from build123d import *

# Parameters (mm, degrees)
SKETCH_1_R          = 23
SKETCH_1_R_2        = 20
EXTRUDE_1_DEPTH     = 51.2
SKETCH_2_R          = 50
SKETCH_2_R_2        = 23
EXTRUDE_2_DEPTH     = 36
EXTRUDE_3_DEPTH     = 15
SKETCH_4_R          = 8
CUT_EXTRUDE_1_DEPTH = 15
SKETCH_5_W          = 2
SKETCH_5_H          = 10
SKETCH_6_R          = 30
CUT_EXTRUDE_2_DEPTH = 2


with BuildPart() as part:
    # Sketch 1 → Extrude 1 (new body)
    with BuildSketch(Plane.XY):
        Circle(SKETCH_1_R)
        Circle(SKETCH_1_R_2, mode=Mode.SUBTRACT)
    extrude(amount=EXTRUDE_1_DEPTH)

    # Sketch 2 → Extrude 2 (add)
    with BuildSketch(Plane.XY):
        Circle(SKETCH_2_R)
        Circle(SKETCH_2_R_2, mode=Mode.SUBTRACT)
    extrude(amount=EXTRUDE_2_DEPTH)

    # Sketch 3 → Extrude 3 (add)
    with BuildSketch(Plane.XY):
        with BuildLine():
            Line((-43.886196735, -23.958333333), (-13.604720988, -79.427083333))
            ThreePointArc((-13.604720988, -79.427083333), (0, -87.5), (13.604720988, -79.427083333))
            Line((13.604720988, -79.427083333), (43.886196735, -23.958333333))
            ThreePointArc((43.886196735, -23.958333333), (0, -50), (-43.886196735, -23.958333333))
        make_face()
        with BuildLine():
            Line((-13.604720988, 79.427083333), (-43.886196735, 23.958333333))
            ThreePointArc((-43.886196735, 23.958333333), (0, 50), (43.886196735, 23.958333333))
            Line((43.886196735, 23.958333333), (13.604720988, 79.427083333))
            ThreePointArc((13.604720988, 79.427083333), (0, 87.5), (-13.604720988, 79.427083333))
        make_face()
    extrude(amount=EXTRUDE_3_DEPTH)

    # Sketch 4 → Cut-Extrude 1 (cut)
    with BuildSketch(Plane.XY):
        with Locations((0, 72)):
            Circle(SKETCH_4_R)
        with Locations((0, -72)):
            Circle(SKETCH_4_R)
    extrude(amount=CUT_EXTRUDE_1_DEPTH, mode=Mode.SUBTRACT)

    # Sketch 5 → Revolve 1 (revolve)
    with BuildSketch(Plane(origin=(0, 0, 0), x_dir=(0, 0, 1), z_dir=(-0.7071067811865488, 0.7071067811865462, 0)), mode=Mode.PRIVATE) as revolve_1_sk:
        with Locations((19, 52)):
            Rectangle(SKETCH_5_W, SKETCH_5_H)
    revolve(revolve_1_sk.sketch.rotate(Axis((-701.140256875, -701.140256875, 18), (0.7071067811865462, 0.7071067811865489, 0)), 90), axis=Axis((-701.140256875, -701.140256875, 18), (0.7071067811865462, 0.7071067811865489, 0)))

    # Sketch 6 → Cut-Extrude 2 (cut)
    with BuildSketch(Plane(origin=(0, 0, 0), x_dir=(-1, 0, 0), z_dir=(0, 0, -1))):
        Circle(SKETCH_6_R)
    extrude(amount=-CUT_EXTRUDE_2_DEPTH, mode=Mode.SUBTRACT)


solid = part.part
Can you work these out from the model? Positions are in its coordinate system, mm. A direction names the side the tool comes from. Round coordinates to 2 decimals unless told otherwise and drop trailing zeros. Order: outer loops, then holes, each group sorted by start corner. A loop starts at its lowest first (then second) coordinate and runs counter-clockwise, first axis right, second up. Notation, with made-up numbers: M 35,53 L 67,53 A16 cw 67,64 Z; hole C 85,-12 d9. An arc over 180 degrees is marked long. Use a Markdown table: item, result.
1) Imagine slicing it at A-A (z = 7). List the corners of the cut face in (x, y) for me, then the cut area to 3 significant figures.
Geometry says:
| item | result |
|---|---|
| outline | M -43.89,-23.96 L -13.6,-79.43 A15.5 ccw 13.6,-79.43 L 43.89,-23.96 A50 ccw 43.89,23.96 L 13.6,79.43 A15.5 ccw -13.6,79.43 L -43.89,23.96 A50 ccw Z; hole C 0,0 d40; hole C 0,-72 d16; hole C 0,72 d16 |
| area | 9,630 mm² |
2) If we mould it in two halves opening along X, with no side actions, what happens to faces 4 (the face through (-2.994, 22.804, 43.494)), 5 (the face through (38, 38, 16)), 6 (the face through (-7, 19, 51.2))? For each: +X half, -X half, draft (parallel to the pull), parting line (faces both ways), or undercut.
Geometry says:
| item | result |
|---|---|
| face 4 | parting line |
| face 5 | undercut |
| face 6 | draft |
3) I'm going to push flat-ended pins straight in: P1, Ø12, axis at x = 1.5, z = 45, coming from the +Y side; P2, Ø1, axis at y = 20.5, z = 13, coming from the +X side; P3, Ø1, axis at x = -9.5, z = 39.5, coming from the +Y side. Where does each tip first touch, or does it pass through?
Geometry says:
| item | result |
|---|---|
| P1 | stops at y = 23 |
| P2 | stops at x = 45.83 |
| P3 | stops at y = 21.17 |
4) Imagine slicing it at D-D (x = 17). List the corners of the cut face in (y, z) for me.
Geometry says:
| item | result |
|---|---|
| outline | M -73.21,0 L -24.72,0 L -24.72,2 L -10.54,2 L -10.54,51.2 L -15.49,51.2 L -15.49,36 L -47.02,36 L -47.02,15 L -73.21,15 Z; M 10.54,2 L 24.72,2 L 24.72,0 L 73.21,0 L 73.21,15 L 47.02,15 L 47.02,36 L 15.49,36 L 15.49,51.2 L 10.54,51.2 Z |
5) Imagine slicing it at C-C (y = 0). List the corners of the cut face in (x, z) for me, then the cut area to 3 significant figures.
Geometry says:
| item | result |
|---|---|
| outline | M -50,0 L -30,0 L -30,2 L -20,2 L -20,51.2 L -23,51.2 L -23,36 L -50,36 Z; M 20,2 L 30,2 L 30,0 L 50,0 L 50,36 L 23,36 L 23,51.2 L 20,51.2 Z |
| area | 2,210 mm² |
6) If I drill on line 1 along Y through (x, z) = (0, 37.5); line 2 along Y through (x, z) = (0, 23); line 3 along Z through (x, y) = (20, 35), over which ranges is the centre line in solid material (lowest first)?
Geometry says:
| item | result |
|---|---|
| line 1 | y = -23 to -20, 20 to 23 |
| line 2 | y = -50 to -20, 20 to 50 |
| line 3 | z = 0 to 36 |
7) On a 3-axis mill with a long thin cutter (end or side, diameter ignored), from which of +Z, -Z, +X, -X, +Y, -Y can I reach the whole of each face in a straight line? I mean faces 1 (the face through (10, -22, 36)), 2 (the face through (28.533, -52.081, 7.395)), 3 (the face through (29.97, 1.32, 0.99)). Say none if no direction works.
Geometry says:
| item | result |
|---|---|
| face 1 | +Z |
| face 2 | +Z, -Z, +X, -Y |
| face 3 | -Z |
8) Imagine slicing it at B-B (x = 0). List the corners of the cut face in (y, z) for me.
Geometry says:
| item | result |
|---|---|
| outline | M -87.5,0 L -80,0 L -80,15 L -87.5,15 Z; M -64,0 L -30,0 L -30,2 L -20,2 L -20,51.2 L -23,51.2 L -23,36 L -50,36 L -50,15 L -64,15 Z; M 20,2 L 30,2 L 30,0 L 64,0 L 64,15 L 50,15 L 50,36 L 23,36 L 23,51.2 L 20,51.2 Z; M 80,0 L 87.5,0 L 87.5,15 L 80,15 Z |
